from build123d import *

# Parameters (mm, degrees)
SKETCH_1_R      = 30
SKETCH_1_R_2    = 1.75
SKETCH_1_W      = 25
SKETCH_1_H      = 40
EXTRUDE_6_DEPTH = 1.5
EXTRUDE_7_DEPTH = 5
SKETCH_1_10_R   = 2
SKETCH_1_10_W   = 7
SKETCH_1_10_H   = 7
EXTRUDE_8_DEPTH = 6
FILLET_3_SIZE   = 1.5
FILLET_4_SIZE   = 1.5
EXTRUDE_9_DEPTH = 5
FILLET_5_SIZE   = 1.5


with BuildPart() as part:
    # 草图1 → 凸台-拉伸6 (new body)
    with BuildSketch(Plane.XY):
        Circle(SKETCH_1_R)
        with Locations((18.25, 0)):
            Circle(SKETCH_1_R_2, mode=Mode.SUBTRACT)
        with Locations((-18.25, 0)):
            Circle(SKETCH_1_R_2, mode=Mode.SUBTRACT)
        Rectangle(SKETCH_1_W, SKETCH_1_H, mode=Mode.SUBTRACT)
    extrude(amount=EXTRUDE_6_DEPTH)

    # 草图1<9> → 凸台-拉伸7 (add)
    with BuildSketch(Plane.XY):
        Polygon((-12.5, 20), (-12.5, 0), (0, 0), (12.5, 0), (12.5, 20), align=None)
    extrude(amount=EXTRUDE_7_DEPTH)

    # 草图1<10> → 凸台-拉伸8 (add)
    with BuildSketch(Plane.XY):
        with Locations((8, -24.5)):
            Circle(SKETCH_1_10_R)
        with Locations((0, -24.5)):
            Rectangle(SKETCH_1_10_W, SKETCH_1_10_H)
        with Locations((-8, -24.5)):
            Circle(SKETCH_1_10_R)
    extrude(amount=-EXTRUDE_8_DEPTH)

    # 圆角3
    # a fillet whose section is not a circle: 1.5 mm, written as the material it takes off along each edge
    with BuildSketch(Plane(origin=(8, -24.5, -6), x_dir=(1, 0, 0), z_dir=(0, -1, 0))) as fillet_3_piece_1:
        with BuildLine():
            Bezier((2, FILLET_3_SIZE), (2, 0), (2 - FILLET_3_SIZE, 0), weights=[1, 1, 1])
            Line((2 - FILLET_3_SIZE, 0), (2, 0))
            Line((2, 0), (2, FILLET_3_SIZE))
        make_face()
    revolve(axis=Axis((8, -24.5, -6), (0, 0, 1)), mode=Mode.SUBTRACT)

    # 圆角4
    # a fillet whose section is not a circle: 1.5 mm, written as the material it takes off along each edge
    with BuildSketch(Plane(origin=(-8, -24.5, -6), x_dir=(1, 0, 0), z_dir=(0, -1, 0))) as fillet_4_piece_1:
        with BuildLine():
            Bezier((2, FILLET_4_SIZE), (2, 0), (2 - FILLET_4_SIZE, 0), weights=[1, 1, 1])
            Line((2 - FILLET_4_SIZE, 0), (2, 0))
            Line((2, 0), (2, FILLET_4_SIZE))
        make_face()
    revolve(axis=Axis((-8, -24.5, -6), (0, 0, 1)), mode=Mode.SUBTRACT)

    # 草图1<11> → 凸台-拉伸9 (add)
    with BuildSketch(Plane.XY):
        Polygon((-12.5, 0), (-12.5, -20), (12.5, -20), (12.5, 0), (0, 0), align=None)
    extrude(amount=EXTRUDE_9_DEPTH)

    # 圆角5
    # a fillet whose section is not a circle: 1.5 mm, written as the material it takes off along each edge
    with BuildSketch(Plane(origin=(16.25, 20, 5), x_dir=(0, -1, 0), z_dir=(-1, 0, 0))) as fillet_5_piece_1:
        with BuildLine():
            Bezier((FILLET_5_SIZE, 0), (0, 0), (0, -FILLET_5_SIZE), weights=[1, 1, 1])
            Line((0, -FILLET_5_SIZE), (0, 0))
            Line((0, 0), (FILLET_5_SIZE, 0))
        make_face()
    extrude(amount=32.5, mode=Mode.SUBTRACT)
    with BuildSketch(Plane(origin=(12.5, 23.75, 5), x_dir=(-1, 0, 0), z_dir=(0, -1, 0)), Plane(origin=(-12.5, -23.75, 5), x_dir=(1, 0, 0), z_dir=(0, 1, 0))) as fillet_5_piece_2:
        with BuildLine():
            Bezier((FILLET_5_SIZE, 0), (0, 0), (0, FILLET_5_SIZE), weights=[1, 1, 1])
            Line((0, FILLET_5_SIZE), (0, 0))
            Line((0, 0), (FILLET_5_SIZE, 0))
        make_face()
    extrude(amount=47.5, mode=Mode.SUBTRACT)
    with BuildSketch(Plane(origin=(-16.25, -20, 5), x_dir=(0, 0, -1), z_dir=(1, 0, 0))) as fillet_5_piece_3:
        with BuildLine():
            Bezier((FILLET_5_SIZE, 0), (0, 0), (0, FILLET_5_SIZE), weights=[1, 1, 1])
            Line((0, FILLET_5_SIZE), (0, 0))
            Line((0, 0), (FILLET_5_SIZE, 0))
        make_face()
    extrude(amount=32.5, mode=Mode.SUBTRACT)


solid = part.part
Geometry: final body of the model. Coordinates: model frame, mm. A direction names the side the tool comes from. Coordinates: 2 decimals unless noted, no trailing zeros. Order: outer loops, then holes, each group sorted by start corner. A loop starts at its lowest first (then second) coordinate and runs counter-clockwise, first axis right, second up.
(1) First-contact query: pin 1 (5 mm diameter, centred on x = -2, z = 3.5, fed in from +Y); pin 2 (3 mm diameter, centred on x = 22, y = -17, fed in from +Z); pin 3 (0.6 mm diameter, centred on y = -8, z = 3, fed in from +X); pin 4 (2 mm diameter, centred on x = 18.25, y = 0, fed in from +Z). Flat tips, straight axial feed; report the tip coordinate or a pass-through.
(2) Section query C-C (y = -1). State how many separate pieces and enclosed holes the cut face has, plus the area to 3 significant figures.
(3) Access query for faces 4 (the face through (0, 20, 2)), 5 (the face through (0, -20, 2)), 6 (the face through (-12.5, 0, 2)), 7 (the face through (0, -28, -3)). Directions: +Z, -Z, +X, -X, +Y, -Y. A direction counts if a zero-diameter tool reaches every point of the face in a straight line with its end or side. Return the directions, or none.
(4) Section query A-A (z = -1.25). Return the cut outline in (x, y), plus the area to 3 significant figures.
(5) Section query B-B (x = 18). Return the cut outline in (y, z), plus the area to 3 significant figures.
(6) Draft query along Y for faces 1 (the face through (0, 0, 0)), 2 (the face through (-29.97, 1.32, 0.74)), 3 (the face through (16.5, 0.08, 0.74)). Return one class per face: pulls with the +Y half, pulls with the -Y half, needs draft (parallel to the pull), parting line crosses it, or undercut.
(7) Material intervals for probe 1 along Y at (x, z) = (-8, 3.75); probe 2 along Z at (x, y) = (-13.5, -23.5); probe 3 along Z at (x, y) = (11, -9), sorted ascending.
(8) Section query D-D (x = -18.25). Return the cut outline in (y, z).
Solution:
1. pin 1: stops at y = 30
1. pin 2: stops at z = 1.5
1. pin 3: stops at x = 12.5
1. pin 4: passes through
2. separate pieces: 3
2. enclosed holes: 0
2. area: 168 mm2
3. face 4: +Z, +X, -X, +Y
3. face 5: +Z, +X, -X, -Y
3. face 6: +Z, -X, +Y, -Y
3. face 7: -Z, +X, -X, -Y
4. outline: circle Ø4 at (-8, -24.5); (-3.5, -28) - (3.5, -28) - (3.5, -21) - (-3.5, -21) - close; circle Ø4 at (8, -24.5)
4. area: 74.1 mm2
5. outline: (-24, 0) - (-1.73, 0) - (-1.73, 1.5) - (-24, 1.5) - close; (1.73, 0) - (24, 0) - (24, 1.5) - (1.73, 1.5) - close
5. area: 66.8 mm2
6. face 1: needs draft
6. face 2: parting line crosses it
6. face 3: undercut
7. probe 1: y = -19.99 to 19.99
7. probe 2: z = 0 to 1.5
7. probe 3: z = 0 to 5
8. outline: (-23.81, 0) - (-1.75, 0) - (-1.75, 1.5) - (-23.81, 1.5) - close; (1.75, 0) - (23.81, 0) - (23.81, 1.5) - (1.75, 1.5) - close
